Geometry check sheet. Reference: drawing and pictorial views, mm from the part's lowest x, y, z. Round coordinates to 2 decimals unless told otherwise and drop trailing zeros. Order: outer loops, then holes, each group sorted by start corner. A loop starts at its lowest first (then second) coordinate and runs counter-clockwise, first axis right, second up.
(1) Thickness scan on probe 1 along X at (y, z) = (22.5, 23.5); probe 2 along Z at (x, y) = (2077.5, 13); probe 3 along Z at (x, y) = (122.5, 13.5). Record the ranges inside material, lowest first.
(2) Sectioned sample at B-B, the plane y = 8.75. Enter the section's corners in (x, z).
(3) Depth check by flat-ended pin: pin 1 (1.5 mm diameter, centred on y = 19, z = 276, fed in from +X); pin 2 (1.5 mm diameter, centred on x = 1867, y = 4.5, fed in from +Z); pin 3 (1 mm diameter, centred on x = 483.5, y = 3, fed in from +Z). Enter the tip coordinate at first touch or a pass-through.
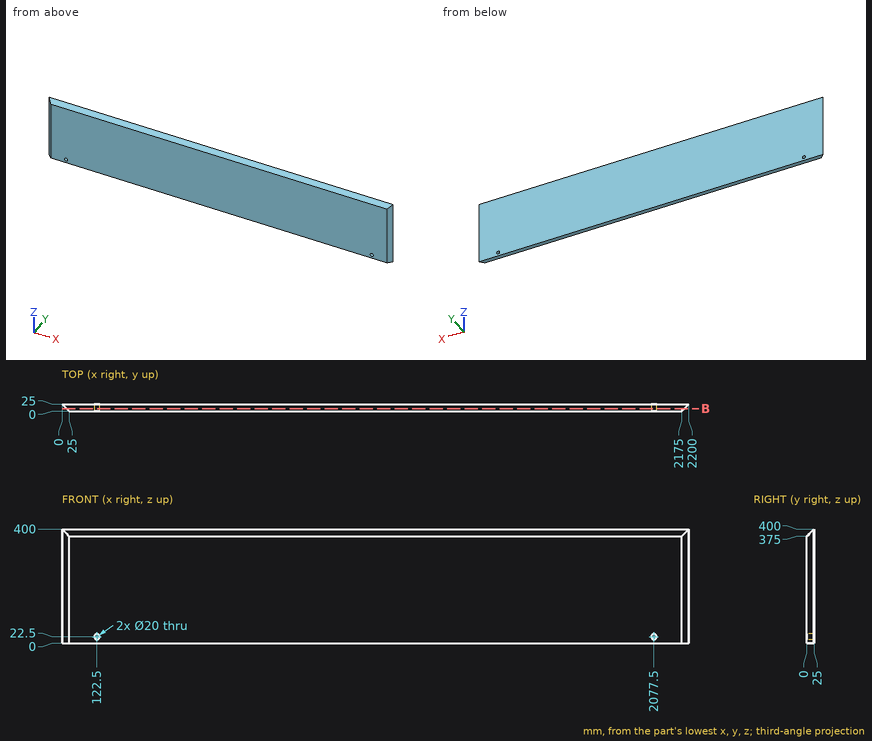
Derived:
1. probe 1: x = 2.5 to 112.55, 132.45 to 2067.55, 2087.45 to 2197.5
1. probe 2: z = 0 to 12.5, 32.5 to 388
1. probe 3: z = 0 to 12.5, 32.5 to 388.5
2. outline: (16.25, 0) - (2183.75, 0) - (2183.75, 383.75) - (16.25, 383.75) - close; hole circle Ø20 at (122.5, 22.5); hole circle Ø20 at (2077.5, 22.5)
3. pin 1: stops at x = 2194.75
3. pin 2: stops at z = 380.25
3. pin 3: stops at z = 378.5
